from build123d import *

# Parameters (mm, degrees)
F0_R     = 3.25
F0_R_2   = 2.25
F1_DEPTH = 51
F0_R_3   = 7.5
F2_DEPTH = 1
F3_R     = 0.49999
F5_R     = 1


# Not quite as in the source:
# - a fillet or chamfer that OpenCascade refuses, or shapes differently, is made with other operations: its cross-section is extruded or revolved along the edge and cut away or added
# - a fillet or chamfer is up to 0.001 mm smaller than in the source, because OpenCascade refuses the exact size


with BuildPart() as f1:
    # F0 (on Top) → F1 (new body)
    with BuildSketch(Plane.XY):
        Circle(F0_R)
        Circle(F0_R_2, mode=Mode.SUBTRACT)
    extrude(amount=F1_DEPTH)

    # F0 (on Top) → F2 (join)
    with BuildSketch(Plane.XY):
        Circle(F0_R_3)
        Circle(F0_R, mode=Mode.SUBTRACT)
    extrude(amount=F2_DEPTH)

    # F3 (radius 0.5 in the source; OpenCascade refuses exactly that, so slightly less here)
    f3_edges = [f1.edges().sort_by_distance(p)[0] for p in [
        (-3.25, 0, 51),
        (-2.25, 0, 51),
    ]]
    fillet(f3_edges, radius=F3_R)

    # F4: fillet of radius 2 on 1 edges, made by hand

    # F4_s1 → F4_t2 (revolve, cut)
    with BuildSketch(Plane.XZ):
        with BuildLine():
            ThreePointArc((7.5, 1), (6.7679491924, 0.2679491924), (5.7679491924, 0))
            Line((5.7679491924, 0), (7.5, 0))
            Line((7.5, 0), (7.5, 1))
        make_face()
    revolve(axis=Axis((0, 0, 0), (0, 0, 1)), mode=Mode.SUBTRACT)

    # F5
    f5_edges = [f1.edges().sort_by_distance(p)[0] for p in [
        (-2.25, 0, 0),
    ]]
    fillet(f5_edges, radius=F5_R)


solid = f1.part
The model under review builds one solid part; all positions refer to its coordinate system, in mm. Give positions to 0.01 mm unless a question says otherwise; leave off trailing zeros. Loops run counter-clockwise (first coordinate to the right, second up) from the corner with the lowest first, then second, coordinate; pieces in that order, holes last. Notation, with made-up numbers: (71.25, 44) -> (121.25, 44) arc R13 cw to (121.25, 54) -> close; hole circle Ø10 at (53.25, 80). An arc over 180 degrees is marked (long way). Answer as a JSON object with one key per item and string values. Group by question number.
Q1. Take a section at C-C (z = 47). Write out the cut boundary in (x, y).
Q2. Draft analysis for pull direction X (two halves, no side actions). For faces 1 (the cylindrical face through (-2.579, -1.978, 25.404)), 2 (the cylindrical face through (-0.29, 2.23, 25.4)), 3 (the flat face through (2, -3, 1)), state which applies: pulls with the +X half, pulls with the -X half, needs draft (parallel to the pull), parting line crosses it, or undercut.
Q3. Insertion check: pin 1 (3 mm diameter, centred on x = 2.5, z = 5, fed in from -Y); pin 2 (8 mm diameter, centred on x = -2, z = 21, fed in from -Y); pin 3 (2 mm diameter, centred on y = -3, z = 40, fed in from -X); pin 4 (1 mm diameter, centred on y = 5.5, z = 27, fed in from -X). Each pin has a flat end and moves straight along its axis. Give the tip position at first contact, or say it passes through.
Q4. Wall thickness on line 1 along Y through (x, z) = (0, 7); line 2 along Z through (x, y) = (-5.75, 0.25); line 3 along X through (y, z) = (-0.5, 9.5): over which ranges is each line inside the solid? List them lowest first.
Answer below:
{
 "1": {"outline": "circle Ø6.5 at (0, 0); hole circle Ø4.5 at (0, 0)"},
 "2": {"face 1": "parting line crosses it", "face 2": "undercut", "face 3": "needs draft"},
 "3": {"pin 1": "stops at y = -3.09", "pin 2": "stops at y = -3.25", "pin 3": "stops at x = -2.56", "pin 4": "passes through"},
 "4": {"line 1": "y = -3.25 to -2.25, 2.25 to 3.25", "line 2": "z = 0 to 1", "line 3": "x = -3.21 to -2.19, 2.19 to 3.21"}
}
